Autodesk Inventor part; units mm, degrees
ref_plane "YZ Plane" through (0, 0, 0) normal (1, 0, 0) x (0, 1, 0)
ref_plane "XZ Plane" through (0, 0, 0) normal (0, 1, 0) x (-1, 0, 0)
ref_plane "XY Plane" through (0, 0, 0) normal (0, 0, 1) x (1, 0, 0)
sketch "Sketch1" plane through (0, 0, 0) normal (0, 0, 1) x (1, 0, 0)
  line L0 (0, 0) -> (88, 0)
  line L1 (88, 0) -> (88, 48)
  line L2 (88, 48) -> (0, 48)
  line L3 (0, 48) -> (0, 0)
  line L4 (18.3534, 5.6399) -> (66.0026, 5.6399)
  line L5 (66.0026, 5.6399) -> (66.0026, 36.8949)
  line L6 (66.0026, 36.8949) -> (18.3534, 36.8949)
  line L7 (18.3534, 36.8949) -> (18.3534, 5.6399)
  dimension "d0" = 88
  dimension "d1" = 48
extrude "Extrusion1" add sketch "Sketch1" along normal blind 12 contours L3 L2 L1 L0 | L7 L6 L5 L4
sketch "Sketch2" plane through (0, 0, 12) normal (0, 0, 1) x (1, 0, 0)
  line L0 (3, 3) -> (85, 3)
  line L1 (85, 3) -> (85, 45)
  line L2 (85, 45) -> (3, 45)
  line L3 (3, 45) -> (3, 3)
  line L4 (88, 48) -> (0, 48)
  line L5 (88, 0) -> (88, 48)
  line L6 (0, 0) -> (88, 0)
  line L7 (0, 48) -> (0, 0)
  dimension "d4" = 3
  dimension "d5" = 3
  dimension "d6" = 3
  dimension "d7" = 3
extrude "Extrusion2" cut sketch "Sketch2" against normal blind 9 contours L3 L2 L1 L0
sketch "Sketch3" plane through (0, 0, 12) normal (0, 0, 1) x (1, 0, 0)
  line L0 (1.5, 46.5) -> (86.5, 46.5)
  line L1 (86.5, 46.5) -> (86.5, 1.5)
  line L2 (86.5, 1.5) -> (1.5, 1.5)
  line L3 (1.5, 1.5) -> (1.5, 46.5)
  line L4 (0, 0) -> (88, 0)
  line L5 (0, 48) -> (0, 0)
  line L6 (88, 0) -> (0, 0)
  line L7 (0, 0) -> (0, 48)
  line L8 (0, 48) -> (88, 48)
  line L9 (88, 48) -> (88, 0)
  dimension "d10" = 1.5
  dimension "d11" = 1.5
  dimension "d12" = 1.5
  dimension "d13" = 1.5
extrude "Extrusion3" cut sketch "Sketch3" against normal blind 1
fillet "Fillet1" radius 2 4 edges at (0, 0, 5.5) (88, 0, 5.5) (88, 48, 5.5) (1.5, 46.5, 11.5)
sketch "Sketch4" plane through (0, 0, 12) normal (0, 0, 1) x (1, 0, 0)
  circle A0 centre (5.5, 24) radius 1
  circle A1 centre (82.5, 24) radius 1
  line L0 (3, 45) -> (85, 45)
  line L1 (3, 3) -> (3, 45)
  line L2 (3, 25.5) -> (5.5, 25.5)
  line L3 (5.5, 25.5) -> (5.5, 22.5)
  line L4 (5.5, 22.5) -> (3, 22.5)
  line L5 (3, 22.5) -> (3, 25.5)
  circle A2 centre (5.5, 24) radius 1.5
  line L6 (85, 45) -> (85, 3)
  line L7 (85, 22.5) -> (82.5, 22.5)
  line L8 (82.5, 22.5) -> (82.5, 25.5)
  line L9 (82.5, 25.5) -> (85, 25.5)
  line L10 (85, 25.5) -> (85, 22.5)
  circle A3 centre (82.5, 24) radius 1.5
  point P0 (0, 0)
  dimension "d17" = 2
  dimension "d18" = 2
  dimension "d19" = 21
  dimension "d20" = 21
  dimension "d21" = 2.5
  dimension "d22" = 3
  dimension "d23" = 1.5
  dimension "d24" = 2.5
  dimension "d25" = 2.5
  dimension "d26" = 3
  dimension "d27" = 1.5
extrude "Extrusion4" add sketch "Sketch4" against normal blind 10
sketch "Sketch5" plane through (0, 0, 12) normal (0, 0, 1) x (1, 0, 0)
  circle A0 centre (5.5, 24) radius 1
  circle A1 centre (82.5, 24) radius 1
  line L0 (3, 25.5) -> (3, 22.5)
  line L1 (3, 22.5) -> (5.5, 22.5)
  line L2 (82.5, 22.5) -> (85, 22.5)
  line L3 (85, 22.5) -> (85, 25.5)
  point P0 (0, 0)
  dimension "d30" = 2
  dimension "d31" = 2
  dimension "d32" = 2.5
  dimension "d33" = 1.5
  dimension "d34" = 1.5
  dimension "d35" = 2.5
extrude "Extrusion5" cut sketch "Sketch5" against normal blind 8
sketch "Sketch6" plane through (0, 0, 3) normal (0, 0, 1) x (1, 0, 0)
  line L0 (35, 45) -> (53, 45)
  line L1 (53, 45) -> (53, 9)
  line L2 (53, 9) -> (35, 9)
  line L3 (35, 9) -> (35, 45)
  line L4 (3, 45) -> (85, 45)
  line L5 (3, 25.5) -> (3, 45)
  point P0 (0, 0)
  dimension "d38" = 18
  dimension "d39" = 36
  dimension "d40" = 0
  dimension "d41" = 32
  dimension "d50" = 82
extrude "Extrusion6" cut sketch "Sketch6" against normal blind 1
sketch "Sketch7" plane through (0, 48, 11) normal (0, 1, 0) x (1, 0, 0)
  line L0 (48.5, 4.8) -> (40.5, 4.8)
  line L1 (40.5, 4.8) -> (40.5, 8)
  line L2 (40.5, 8) -> (48.5, 8)
  line L3 (48.5, 8) -> (48.5, 4.8)
  line L4 (86, 11) -> (0, 11)
  line L5 (86, 11) -> (86, 0)
  dimension "d44" = 8
  dimension "d45" = 3.2
  dimension "d46" = 3
  dimension "d47" = 37.5
extrude "Extrusion7" cut sketch "Sketch7" against normal blind 4
sketch "Sketch8" plane through (0, 48, 11) normal (0, 1, 0) x (1, 0, 0)
  line L0 (50.5, 9.5) -> (38.5, 9.5)
  line L1 (38.5, 9.5) -> (38.5, 3.3)
  line L2 (38.5, 3.3) -> (50.5, 3.3)
  line L3 (50.5, 3.3) -> (50.5, 9.5)
  line L4 (48.5, 8) -> (48.5, 4.8)
  line L5 (40.5, 4.8) -> (40.5, 8)
  line L6 (48.5, 4.8) -> (40.5, 4.8)
  line L7 (40.5, 8) -> (48.5, 8)
  point P0 (0, 11)
  dimension "d51" = 2
  dimension "d52" = 2
  dimension "d53" = 1.5
  dimension "d54" = 1.5
extrude "Extrusion8" cut sketch "Sketch8" against normal blind 1
properties part number "Base"
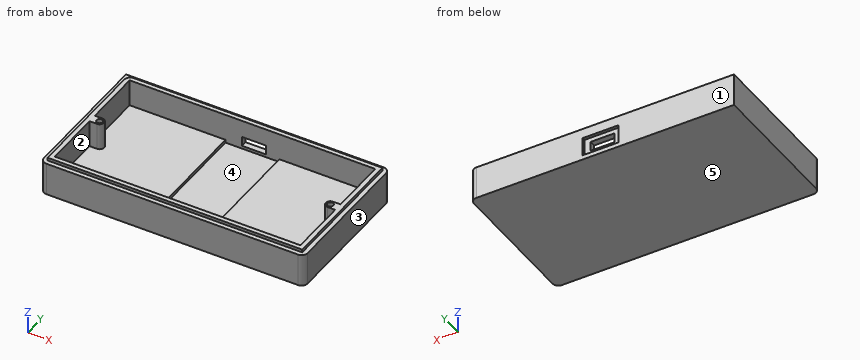
Here's how the part is built. I have some questions about the finished solid (model axes, mm). Face numbers are marked on the shaded views. A direction names the side the tool comes from. Coordinates: 2 decimals unless noted, no trailing zeros. Write each loop counter-clockwise with the first axis right and the second up, starting at its lowest first coordinate (ties: lowest second). Pieces come first, ordered by that corner, then holes.
Item 1: On a 3-axis mill with a long thin cutter (end or side, diameter ignored), from which of +Z, -Z, +X, -X, +Y, -Y can I reach the whole of each face in a straight line? I mean the marked faces 1 and 2. Say none if no direction works.
Item 2: If we mould it in two halves opening along X, with no side actions, what happens to the marked faces 3, 4 and 5? For each: +X half, -X half, draft (parallel to the pull), parting line (faces both ways), or undercut.
Item 3: I want a section at D-D on y = 8. Write out the boundary of the cut face in (x, z).
Item 4: I want a section at B-B on z = 9.25. Write out the boundary of the cut face in (x, y).
Item 5: Will these pins go through, and if not, where does the flat tip stop? pin 1 (1.5 mm diameter, centred on x = 20.5, y = 41, fed in from -Z); pin 2 (3 mm diameter, centred on x = 48.5, y = 24, fed in from +Z); pin 3 (0.8 mm diameter, centred on x = 41, z = 2.5, fed in from +Y); pin 4 (0.5 mm diameter, centred on y = 47.5, z = 3.5, fed in from +X).
Item 6: I want a section at A-A on y = 42.5. Write out the boundary of the cut face in (x, z).
Item 7: If I drill on line 1 (Y direction, x = 82.5, z = 7.5); line 2 (Y direction, x = 66.5, z = 8.75); line 3 (X direction, y = 13, z = 4.5), over which ranges is the centre line in solid material (lowest first)?
Item 8: I want a section at C-C on x = 70. Write out the boundary of the cut face in (y, z), and give its area (3 significant figures).
Findings below:
1. face 1: +Z, -Z, +X, -X, +Y
1. face 2: +Z
2. face 3: +X half
2. face 4: undercut
2. face 5: draft
3. outline: (0, 0) - (88, 0) - (88, 11) - (86.5, 11) - (86.5, 12) - (85, 12) - (85, 3) - (3, 3) - (3, 12) - (1.5, 12) - (1.5, 11) - (0, 11) - close
4. outline: (0, 2) arc R2 ccw to (2, 0) - (86, 0) arc R2 ccw to (88, 2) - (88, 46) arc R2 ccw to (86, 48) - (0, 48) - close; hole (3, 3) - (85, 3) - (85, 22.5) - (82.5, 22.5) arc R1.5 cw to (82.5, 25.5) - (85, 25.5) - (85, 45) - (3, 45) - (3, 25.5) - (5.5, 25.5) arc R1.5 cw to (5.5, 22.5) - (3, 22.5) - close; hole circle Ø2 at (5.5, 24); hole circle Ø2 at (82.5, 24)
5. pin 1: stops at z = 0
5. pin 2: stops at z = 2
5. pin 3: stops at y = 47
5. pin 4: stops at x = 87.56
6. outline: (0, 0) - (88, 0) - (88, 11) - (86.5, 11) - (86.5, 12) - (85, 12) - (85, 3) - (53, 3) - (53, 2) - (35, 2) - (35, 3) - (3, 3) - (3, 12) - (1.5, 12) - (1.5, 11) - (0, 11) - close
7. line 1: y = 0 to 3, 22.5 to 23, 25 to 25.5, 45 to 48
7. line 2: y = 0 to 3, 45 to 48
7. line 3: x = 0 to 3, 85 to 88
8. outline: (0, 0) - (48, 0) - (48, 11) - (46.5, 11) - (46.5, 12) - (45, 12) - (45, 3) - (3, 3) - (3, 12) - (1.5, 12) - (1.5, 11) - (0, 11) - close
8. area: 195 mm2
